```python
from build123d import *

# Parameters (mm, degrees)
SKETCH1_R           = 4.075
SKETCH1_R_2         = 5.075
BOSS_EXTRUDE1_DEPTH = 1
BOSS_EXTRUDE3_START = 4
BOSS_EXTRUDE3_DEPTH = 4
FILLET2_R           = 0.75
SKETCH4_R           = 6.5
SKETCH4_R_2         = 4.075
SKETCH4_R_3         = 5.075
BOSS_EXTRUDE4_DEPTH = 10


with BuildPart() as part:
    # Sketch1 → Boss-Extrude1 (new body)
    with BuildSketch(Plane(origin=(0, 0, 0), x_dir=(1, 0, 0), z_dir=(0, 1, 0))):
        with BuildLine():
            Line((14.4, -14.4), (14.4, 116.534474513))
            ThreePointArc((14.4, 116.534474513), (5.510641426, 129.838339781), (-10.182337649, 126.716812162))
            Line((-10.182337649, 126.716812162), (-126.716812162, 10.182337649))
            ThreePointArc((-126.716812162, 10.182337649), (-129.838339781, -5.510641426), (-116.534474513, -14.4))
            Line((-116.534474513, -14.4), (14.4, -14.4))
        make_face()
        with Locations(Location((-116.534474513, 0, 0), (0, 0, 270))):
            Circle(SKETCH1_R, mode=Mode.SUBTRACT)
        with Locations(Location((0, 116.534474513, 0), (0, 0, 270))):
            Circle(SKETCH1_R, mode=Mode.SUBTRACT)
        with Locations(Location((0, 0, 0), (0, 0, 270))):
            Circle(SKETCH1_R, mode=Mode.SUBTRACT)
        with Locations(Location((-91.907842371, 24.626632142, 0), (0, 0, 270))):
            Circle(SKETCH1_R_2, mode=Mode.SUBTRACT)
        with Locations(Location((-24.626632142, 91.907842371, 0), (0, 0, 270))):
            Circle(SKETCH1_R_2, mode=Mode.SUBTRACT)
    extrude(amount=BOSS_EXTRUDE1_DEPTH)

    # Sketch3 → Boss-Extrude3 (add)
    with BuildSketch(Plane.XZ.offset(BOSS_EXTRUDE3_START)):
        with BuildLine():
            Line((12.4, 12.4), (12.4, -123.8556766))
            ThreePointArc((12.4, -123.8556766), (13.891004283, -120.329207705), (14.4, -116.534474513))
            Line((14.4, -116.534474513), (14.4, 14.4))
            Line((14.4, 14.4), (-116.534474513, 14.4))
            ThreePointArc((-116.534474513, 14.4), (-120.329207705, 13.891004283), (-123.8556766, 12.4))
            Line((-123.8556766, 12.4), (12.4, 12.4))
        make_face()
    extrude(amount=-BOSS_EXTRUDE3_DEPTH)

    # Fillet2
    fillet2_edges = [part.edges().sort_by_distance(p)[0] for p in [
        (-123.8556766, -2, 12.4),
        (12.4, -2, -123.8556766),
    ]]
    fillet(fillet2_edges, radius=FILLET2_R)

    # Sketch4 → Boss-Extrude4 (add)
    # profile 1 of 5: a face of its own
    with BuildSketch(Plane(origin=(0, 1, 0), x_dir=(1, 0, 0), z_dir=(0, 1, 0))):
        with Locations(Location((-116.534474513, 0, 0), (0, 0, 270))):
            Circle(SKETCH4_R)
        with Locations(Location((-116.534474513, 0, 0), (0, 0, 270))):
            Circle(SKETCH4_R_2, mode=Mode.SUBTRACT)
    # profile 2 of 5: a face of its own
    with BuildSketch(Plane(origin=(0, 1, 0), x_dir=(1, 0, 0), z_dir=(0, 1, 0))):
        with Locations(Location((0, 116.534474513, 0), (0, 0, 270))):
            Circle(SKETCH4_R)
        with Locations(Location((0, 116.534474513, 0), (0, 0, 270))):
            Circle(SKETCH4_R_2, mode=Mode.SUBTRACT)
    # profile 3 of 5: a face of its own
    with BuildSketch(Plane(origin=(0, 1, 0), x_dir=(1, 0, 0), z_dir=(0, 1, 0))):
        with Locations(Location((-91.907842371, 24.626632142, 0), (0, 0, 270))):
            Circle(SKETCH4_R)
        with Locations(Location((-91.907842371, 24.626632142, 0), (0, 0, 270))):
            Circle(SKETCH4_R_3, mode=Mode.SUBTRACT)
    # profile 4 of 5: a face of its own
    with BuildSketch(Plane(origin=(0, 1, 0), x_dir=(1, 0, 0), z_dir=(0, 1, 0))):
        with Locations(Location((-24.626632142, 91.907842371, 0), (0, 0, 270))):
            Circle(SKETCH4_R)
        with Locations(Location((-24.626632142, 91.907842371, 0), (0, 0, 270))):
            Circle(SKETCH4_R_3, mode=Mode.SUBTRACT)
    # profile 5 of 5: a face of its own
    with BuildSketch(Plane(origin=(0, 1, 0), x_dir=(1, 0, 0), z_dir=(0, 1, 0))):
        with Locations(Location((0, 0, 0), (0, 0, 270))):
            Circle(SKETCH4_R)
        with Locations(Location((0, 0, 0), (0, 0, 270))):
            Circle(SKETCH4_R_2, mode=Mode.SUBTRACT)
    extrude(amount=BOSS_EXTRUDE4_DEPTH)


solid = part.part
```
Read the model definition and answer for the solid it produces. Units are mm, in the model's axes. A direction names the side the tool comes from. Round coordinates to 2 decimals unless told otherwise and drop trailing zeros. Write each loop counter-clockwise with the first axis right and the second up, starting at its lowest first coordinate (ties: lowest second). Pieces come first, ordered by that corner, then holes. Notation, with made-up numbers: (76, 1.5) -> (103, 1.5) arc R20 ccw to (103, 38.5) -> close; hole circle Ø4 at (63.25, -5.5). An arc over 180 degrees is marked (long way). Answer in a Markdown table with one row per item. Add a question column.
1) Which of the six approach directions +Z, -Z, +X, -X, +Y, -Y give full straight-line access (tool end or side, diameter ignored) to faces 1 (the face through (12.4, -2, -53)), 2 (the face through (-19.15, 5.93, -88.41)), 3 (the face through (-3, 11, -120))?
2) Find section A-A, the plane z = 0. Determine the outline of the cut face in (x, y) (3 decimals).
3) Given P1, Ø1.5, axis at x = -71.5, y = 0.5, coming from the -Z side; P2, Ø8, axis at x = -72.5, y = 4, coming from the -Z side; P3, Ø6, axis at x = -58.5, z = -63, coming from the -Y side, each flat-ended and moving along its own axis, determine where each tip first touches the part or whether it passes through.
4) Find section C-C, the plane y = 8. State how many separate pieces and enclosed holes the cut face has, and give its area (3 significant figures).
5) Determine the mould class of faces 4 (the face through (-2.49, 5.93, -110.53)), 5 (the face through (-26.57, 5.42, -87.22)), 6 (the face through (-96, 11, -28)), 7 (the face through (-50, -2, 14.4)) for opening direction Z: pulls with the +Z half, pulls with the -Z half, needs draft (parallel to the pull), parting line crosses it, or undercut.
6) Consider line 1 (X direction, y = 7.5, z = 0) (3 decimals); line 2 (Y direction, x = -82, z = -31); line 3 (Y direction, x = -86, z = -27). Determine where each line is inside the solid, lowest interval first.
7) Find section D-D, the plane x = -88.5. Determine the outline of the cut face in (y, z).
8) Find section B-B, the plane x = 0. Determine the outline of the cut face in (y, z) (3 decimals).
Findings below:
| question | item | result |
|---|---|---|
| 1 | face 1 | -Z, -X, -Y |
| 1 | face 2 | +Y |
| 1 | face 3 | +Z, -Z, +X, -X, +Y |
| 2 | outline | (-130.934, 0) -> (-120.609, 0) -> (-120.609, 11) -> (-123.034, 11) -> (-123.034, 1) -> (-130.934, 1) -> close; (-112.459, 0) -> (-4.075, 0) -> (-4.075, 11) -> (-6.5, 11) -> (-6.5, 1) -> (-110.034, 1) -> (-110.034, 11) -> (-112.459, 11) -> close; (4.075, 0) -> (12.4, 0) -> (12.4, -4) -> (14.4, -4) -> (14.4, 1) -> (6.5, 1) -> (6.5, 11) -> (4.075, 11) -> close |
| 3 | P1 | z = -66.15 |
| 3 | P2 | z = -67.04 |
| 3 | P3 | y = 0 |
| 4 | separate pieces | 5 |
| 4 | enclosed holes | 5 |
| 4 | area | 345 mm² |
| 5 | face 4 | undercut |
| 5 | face 5 | undercut |
| 5 | face 6 | needs draft |
| 5 | face 7 | pulls with the +Z half |
| 6 | line 1 | -123.034 to -120.609, -112.459 to -110.034, -6.5 to -4.075, 4.075 to 6.5 |
| 6 | line 2 | 0 to 1 |
| 6 | line 3 | 0 to 11 |
| 7 | outline | (-4, 12.4) -> (0, 12.4) -> (0, -20.87) -> (11, -20.87) -> (11, -19.09) -> (1, -19.09) -> (1, 14.4) -> (-4, 14.4) -> close; (0, -48.4) -> (1, -48.4) -> (1, -30.16) -> (11, -30.16) -> (11, -28.39) -> (0, -28.39) -> close |
| 8 | outline | (-4, 12.4) -> (0, 12.4) -> (0, 4.075) -> (11, 4.075) -> (11, 6.5) -> (1, 6.5) -> (1, 14.4) -> (-4, 14.4) -> close; (0, -130.934) -> (1, -130.934) -> (1, -123.034) -> (11, -123.034) -> (11, -120.609) -> (0, -120.609) -> close; (0, -112.459) -> (11, -112.459) -> (11, -110.034) -> (1, -110.034) -> (1, -6.5) -> (11, -6.5) -> (11, -4.075) -> (0, -4.075) -> close |
